Autodesk Inventor part; units mm, degrees
ref_plane "YZ Plane" through (0, 0, 0) normal (1, 0, 0) x (0, 1, 0)
ref_plane "XZ Plane" through (0, 0, 0) normal (0, 1, 0) x (-1, 0, 0)
ref_plane "XY Plane" through (0, 0, 0) normal (0, 0, 1) x (1, 0, 0)
sketch "Sketch1" plane through (0, 0, 0) normal (0, 1, 0) x (-1, 0, 0)
  line L0 (-98.3907, 29.7008) -> (54.0093, 29.7008)
  line L1 (54.0093, 29.7008) -> (54.0093, -71.8992)
  line L2 (54.0093, -71.8992) -> (-98.3907, -71.8992)
  line L3 (-98.3907, -71.8992) -> (-98.3907, 29.7008)
  point P0 (0, 0)
  dimension "d0" = 152.4
  dimension "d1" = 101.6
extrude "Extrusion1" add sketch "Sketch1" along normal blind 31.75
sketch "Sketch2" plane through (98.3907, 0, 29.7008) normal (1, 0, 0) x (0, 0, -1)
  line L0 (0, 31.75) -> (101.6, 31.75)
  line L1 (2.6537, 35.2563) -> (7.0386, 2.4572)
  line L2 (7.0386, 2.4572) -> (9.3017, 2.7597)
  line L3 (9.3017, 2.7597) -> (10.7219, 35.2563)
  line L4 (10.7219, 35.2563) -> (2.6537, 35.2563)
  point P0 (29.7008, 0)
extrude "Extrusion2" cut sketch "Sketch2" against normal up to next
pattern_linear "Rectangular Pattern1" count 8 spacing 12.7 along (0, 0, -1) of "Extrusion2"
properties part number "HeatSink"
Read the model definition and answer for the solid it produces. Units are mm, in the model's axes. A direction names the side the tool comes from. Round coordinates to 2 decimals unless told otherwise and drop trailing zeros.
Q1. A tool of negligible diameter and unlimited length cuts with its end or side. For faces 1 (the face through (23, 31.75, 28)), 2 (the face through (23.257, 17.052, -56.426)), from which of +Z, -Z, +X, -X, +Y, -Y can it reach the whole face along a straight path? Write none if from no direction.
Values:
face 1: +Z, -Z, +X, -X, +Y
face 2: +X, -X, +Y
Q2. A straight line is drawn through the part: line 1 (Y direction, x = 43, z = 8). Find the intervals that lie inside material, in ascending order.
Values:
line 1: y = 0 to 2.72
Q3. A flat-ended cylindrical pin translates along its axis: P1, Ø3, axis at x = 31.5, z = -26, coming from the -Y side. Find the tip coordinate at first contact, or state that the pin passes through.
Values:
P1: stops at y = 0
Q4. The mould has two halves that part along Z. Classify faces 3 (the face through (23, 31.75, -9)), 4 (the face through (23.257, 17.309, -26.152)), 5 (the face through (23, 16, 29.701)), 6 (the face through (23.257, 17.309, -13.452)): released by +Z, released by -Z, zero draft, split by the parting line, or undercut.
Values:
face 3: zero draft
face 4: undercut
face 5: released by +Z
face 6: undercut
Q5. Find section A-A on y = 5. State how many separate pieces and enclosed holes the cut face has, and give its area (3 significant figures).
Values:
separate pieces: 9
enclosed holes: 0
area: 12,200 mm2
